The listing builds one solid part. Answer for the finished solid, in the listing's coordinates (mm). A direction names the side the tool comes from. Round coordinates to 2 decimals unless told otherwise and drop trailing zeros. Loops run counter-clockwise (first coordinate to the right, second up) from the corner with the lowest first, then second, coordinate; pieces in that order, holes last. Notation, with made-up numbers: M -24.75,56 L 2.25,56 A13 ccw 2.25,77 Z; hole C 26.25,69.25 d5. An arc over 180 degrees is marked long. Answer as a JSON object with one key per item and string values.
```python
from build123d import *

# Parameters (mm, degrees)
F0_R     = 20.426716
F1_DEPTH = 25
F3_DEPTH = 25
F5_D     = 5


with BuildPart() as f1:
    # F0 (on Top) → F1 (new body)
    with BuildSketch(Plane.XY):
        Circle(F0_R)
    extrude(amount=F1_DEPTH)

    # F2 (on face) → F3 (join)
    with BuildSketch(Plane.XY.offset(25)):
        Polygon((-9.159605, -8.859223), (12.427566, -12.093626), (0, 0), (3.715735, 17.731052), (-17.018216, 4.805511), align=None)
    extrude(amount=F3_DEPTH)

    # F5 (through all)
    with Locations(Plane(origin=(0, 0, 0), x_dir=(1, 0, 0), z_dir=(0, 0, -1))):
        with Locations((-11.890458, 0), (13.805311, 0)):
            Hole(F5_D / 2)


solid = f1.part
```
Item 1: Flat-ended cylindrical pins translate along their axes: P1, Ø4.5, axis at x = -11.89, y = 0, coming from the -Z side; P2, Ø12, axis at x = 10.5, z = 9.5, coming from the +Y side; P3, Ø12, axis at y = 9, z = 14.5, coming from the -X side; P4, Ø5, axis at x = -3, z = 19.5, coming from the -Y side. Find the tip coordinate at first contact, or state that the pin passes through.
Values follow:
{"P1": "through", "P2": "y = 19.92", "P3": "x = -20.21", "P4": "y = -20.42"}
Item 2: The part is cut by section C-C (z = 45). Give the vertices of the cut face in (x, y), then the cut area to 3 significant figures.
Values follow:
{"outline": "M -17.02,4.81 L -14.38,0.22 A2.5 cw long -12.95,-2.26 L -9.16,-8.86 L 12.43,-12.09 L 0,0 L 3.72,17.73 Z", "area": "349 mm^2"}
Item 3: The part is cut by section B-B (y = -1). Give the vertices of the cut face in (x, z), then the cut area to 3 significant figures.
Values follow:
{"outline": "M -20.4,0 L -14.18,0 L -14.18,25 L -20.4,25 Z; M -9.6,0 L 11.51,0 L 11.51,25 L 1.03,25 L 1.03,50 L -9.6,50 Z; M 16.1,0 L 20.4,0 L 20.4,25 L 16.1,25 Z", "area": "1,060 mm^2"}
Item 4: Determine the mould class of faces 1 (the face through (1.483, -10.454, 37.325)), 2 (the face through (1.83, 8.74, 37.33)), 3 (the face through (-6.506, 11.359, 37.325)) for opening direction Y: released by +Y, released by -Y, zero draft, split by the parting line, or undercut.
Values follow:
{"face 1": "released by -Y", "face 2": "undercut", "face 3": "released by +Y"}
Item 5: The part is cut by section A-A (x = -11). Give the vertices of the cut face in (y, z), then the cut area to 3 significant figures.
Values follow:
{"outline": "M -17.21,0 L -2.34,0 L -2.34,50 L -5.66,50 L -5.66,25 L -17.21,25 Z; M 2.34,0 L 17.21,0 L 17.21,25 L 8.56,25 L 8.56,50 L 2.34,50 Z", "area": "982 mm^2"}
Item 6: Straight lines are drawn through the part: line 1 (Z direction, x = -2, y = -12.5); line 2 (Y direction, x = -14, z = 13.5); line 3 (X direction, y = 1, z = 32.5). For each, find the intervals that lie inside material, in ascending order.
Values follow:
{"line 1": "0 to 25", "line 2": "-14.87 to -1.34, 1.34 to 14.87", "line 3": "-14.83 to -14.18, -9.6 to 0.21"}
Item 7: The part is cut by section D-D (y = 12.5). Give the vertices of the cut face in (x, z), then the cut area to 3 significant figures.
Values follow:
{"outline": "M -16.16,0 L 16.16,0 L 16.16,25 L 2.62,25 L 2.62,50 L -4.68,50 L -4.68,25 L -16.16,25 Z", "area": "990 mm^2"}
Item 8: Which of the six approach directions +Z, -Z, +X, -X, +Y, -Y give full straight-line access (tool end or side, diameter ignored) to faces 4 (the face through (6.3, -6.13, 37.33)), 5 (the face through (-9.907, 1.521, 25.35)), 6 (the face through (-11.083, -5.515, 37.325))?
Values follow:
{"face 4": "+Z, +X", "face 5": "+Z, -Z", "face 6": "+Z, -X, -Y"}
